Verification items for this drawing (mm, ordinates from the low corner). Round coordinates to 2 decimals unless told otherwise and drop trailing zeros. Order: outer loops, then holes, each group sorted by start corner. A loop starts at its lowest first (then second) coordinate and runs counter-clockwise, first axis right, second up. Notation, with made-up numbers: (-30, 80.25) -> (-5, 80.25) arc R20 ccw to (-5, 112.25) -> close; hole circle Ø7 at (10, 37). An arc over 180 degrees is marked (long way). Answer in a Markdown table with one row per item.
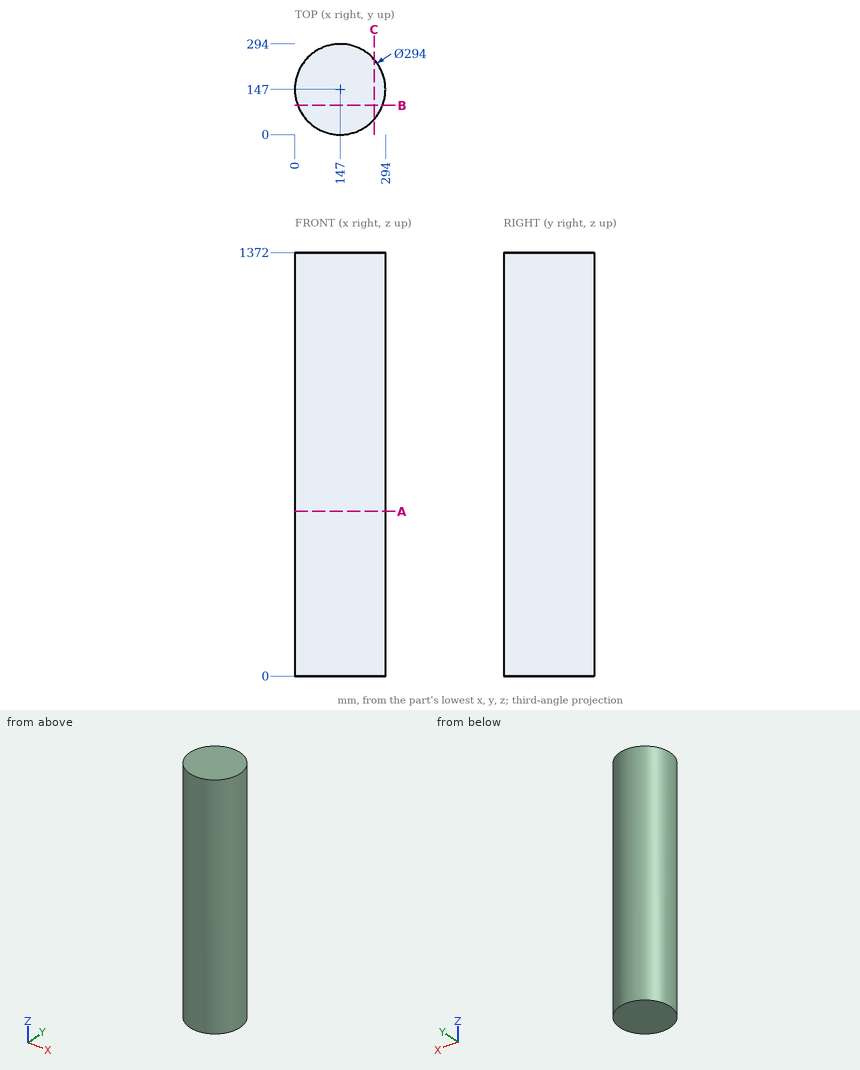
Item 1: Cross-section at A-A (z = 533.5). Record the boundary of the cut face in (x, y).
Result sheet:
| item | result |
|---|---|
| outline | circle Ø294 at (147, 147) |
Item 2: Cross-section at C-C (x = 257). Record the boundary of the cut face in (y, z), and give its area (3 significant figures).
Result sheet:
| item | result |
|---|---|
| outline | (49.49, 0) -> (244.51, 0) -> (244.51, 1372) -> (49.49, 1372) -> close |
| area | 268,000 mm^2 |
Item 3: Depth check by flat-ended pin: P1, Ø2, axis at y = 90.5, z = 774, coming from the -X side; P2, Ø4, axis at x = 230, z = 862, coming from the +Y side; P3, Ø10, axis at x = 85, z = 292, coming from the -Y side. Enter the tip coordinate at first touch or a pass-through.
Result sheet:
| item | result |
|---|---|
| P1 | stops at x = 10.88 |
| P2 | stops at y = 269.67 |
| P3 | stops at y = 11.5 |
Item 4: Scan lines: line 1 (X direction, y = 153, z = 1162); line 2 (Y direction, x = 210.5, z = 1150); line 3 (Y direction, x = 54.5, z = 349). Record each from-to range of solid material in increasing order. Write a range as [from, to].
Result sheet:
| item | result |
|---|---|
| line 1 | x = [0.12, 293.88] |
| line 2 | y = [14.42, 279.58] |
| line 3 | y = [32.75, 261.25] |
Item 5: Cross-section at B-B (y = 95). Record the boundary of the cut face in (x, z), and give its area (3 significant figures).
Result sheet:
| item | result |
|---|---|
| outline | (9.5, 0) -> (284.5, 0) -> (284.5, 1372) -> (9.5, 1372) -> close |
| area | 377,000 mm^2 |
